Study the drawing (mm; zero at the part's minimum x, y, z) and answer. Give positions to 0.01 mm unless a question says otherwise; leave off trailing zeros. Write each loop counter-clockwise with the first axis right and the second up, starting at its lowest first coordinate (ties: lowest second). Pieces come first, ordered by that corner, then holes.
1) Find section C-C (z = 38.1). Determine the outline of the cut face in (x, y) (3 decimals).
2) Given pin 1 Ø1.9 at (x, y) = (41.5, 5) entering from -Z, flat-ended and moving along its own axis, determine where the tip first touches the part or whether it passes through.
3) Find section A-A (x = 25.4). Determine the outline of the cut face in (y, z) (3 decimals).
4) Straight lines are drawn through the part: probe 1 along Z at (x, y) = (25.4, 8) (3 decimals); probe 2 along X at (y, z) = (5.25, 8.5); probe 3 along X at (y, z) = (7.25, 38.1) (3 decimals). For each, find the intervals that lie inside material, in ascending order.
5) Find section D-D (y = 1.25). Determine the outline of the cut face in (x, z) (3 decimals).
6) Determine the mould class of the marked faces 1, 2 and 3 for opening direction X: pulls with the +X half, pulls with the -X half, needs draft (parallel to the pull), parting line crosses it, or undercut.
7) Find section B-B (y = 6.35). Determine the outline of the cut face in (x, z) (3 decimals).
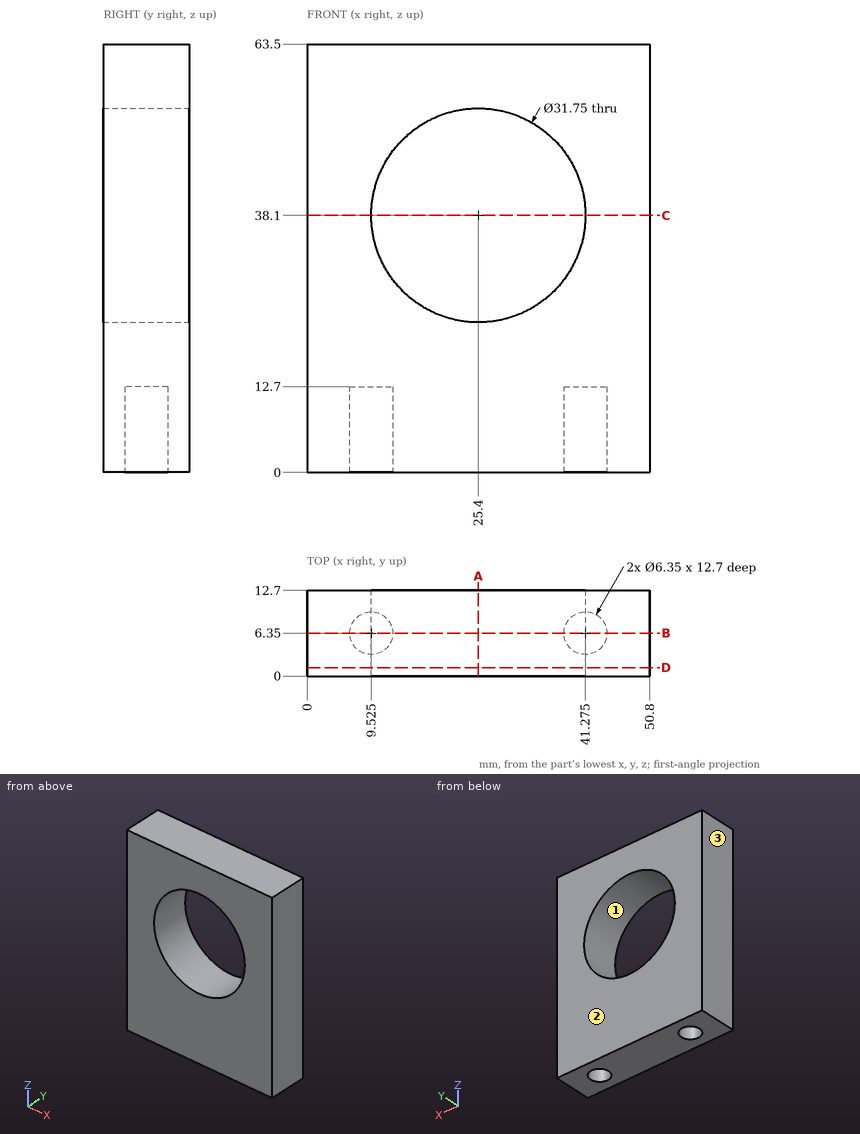
Results:
1. outline: (0, 0) - (9.525, 0) - (9.525, 12.7) - (0, 12.7) - close; (41.275, 0) - (50.8, 0) - (50.8, 12.7) - (41.275, 12.7) - close
2. pin 1: stops at z = 12.7
3. outline: (0, 0) - (12.7, 0) - (12.7, 22.225) - (0, 22.225) - close; (0, 53.975) - (12.7, 53.975) - (12.7, 63.5) - (0, 63.5) - close
4. probe 1: z = 0 to 22.225, 53.975 to 63.5
4. probe 2: x = 0 to 6.55, 12.5 to 38.3, 44.25 to 50.8
4. probe 3: x = 0 to 9.525, 41.275 to 50.8
5. outline: (0, 0) - (50.8, 0) - (50.8, 63.5) - (0, 63.5) - close; hole circle Ø31.75 at (25.4, 38.1)
6. face 1: undercut
6. face 2: needs draft
6. face 3: pulls with the -X half
7. outline: (0, 0) - (6.35, 0) - (6.35, 12.7) - (12.7, 12.7) - (12.7, 0) - (38.1, 0) - (38.1, 12.7) - (44.45, 12.7) - (44.45, 0) - (50.8, 0) - (50.8, 63.5) - (0, 63.5) - close; hole circle Ø31.75 at (25.4, 38.1)
